Geometry: see drawing. Coordinates: mm, zero at the bounding-box minimum. A direction names the side the tool comes from. Give positions to 0.01 mm unless a question says otherwise; leave off trailing zeros. Loops run counter-clockwise (first coordinate to the right, second up) from the corner with the lowest first, then second, coordinate; pieces in that order, holes last. Notation, with made-up numbers: M 38,70.25 L 48,70.25 A5 cw 48,76.25 Z; hole C 11,36 d1. An arc over 180 degrees is marked long. Answer in a Markdown table with one row per item.
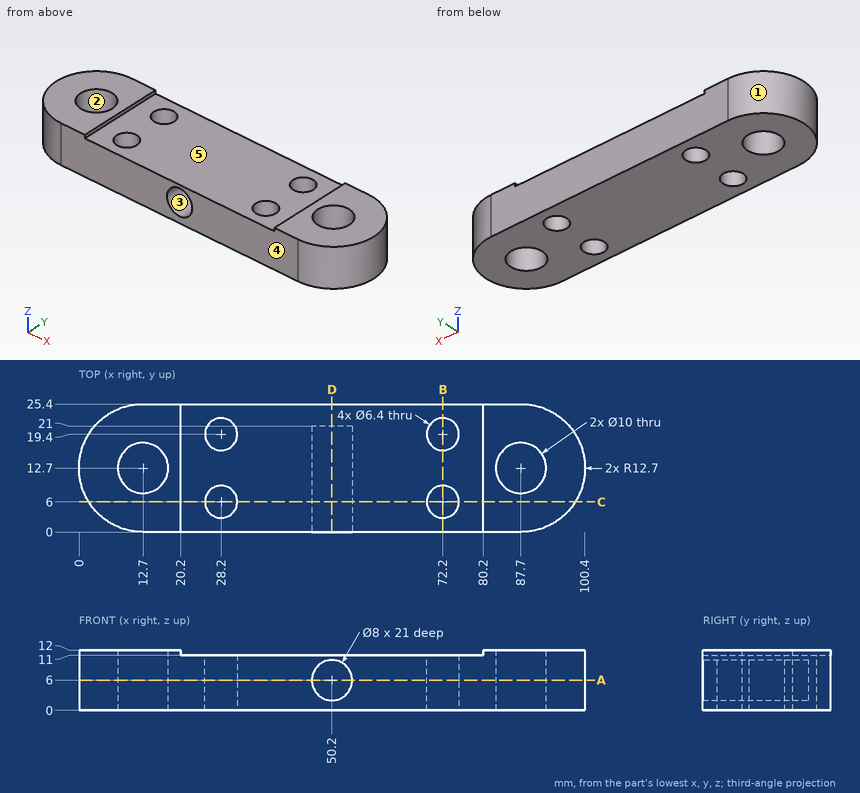
1) Section C-C, the plane y = 6. Return loops of the section in (x, z), then the cut area to 3 significant figures.
Reply:
| item | result |
|---|---|
| outline | M 1.91,0 L 25,0 L 25,11 L 20.2,11 L 20.2,12 L 1.91,12 Z; M 31.4,0 L 69,0 L 69,11 L 31.4,11 Z; M 75.4,0 L 98.49,0 L 98.49,12 L 80.2,12 L 80.2,11 L 75.4,11 Z; hole C 50.2,6 d8 |
| area | 908 mm² |
2) Section A-A, the plane z = 6. Return loops of the section in (x, y), then the cut area to 3 significant figures.
Reply:
| item | result |
|---|---|
| outline | M 12.7,0 L 46.2,0 L 46.2,21 L 54.2,21 L 54.2,0 L 87.7,0 A12.7 ccw 87.7,25.4 L 12.7,25.4 A12.7 ccw Z; hole C 12.7,12.7 d10; hole C 28.2,6 d6.4; hole C 28.2,19.4 d6.4; hole C 72.2,6 d6.4; hole C 72.2,19.4 d6.4; hole C 87.7,12.7 d10 |
| area | 1,960 mm² |
3) Section B-B, the plane x = 72.2. Return loops of the section in (y, z), then the cut area to 3 significant figures.
Reply:
| item | result |
|---|---|
| outline | M 0,0 L 2.8,0 L 2.8,11 L 0,11 Z; M 9.2,0 L 16.2,0 L 16.2,11 L 9.2,11 Z; M 22.6,0 L 25.4,0 L 25.4,11 L 22.6,11 Z |
| area | 139 mm² |
4) Set-up query: the marked faces 4 and 5. Return all of +Z, -Z, +X, -X, +Y, -Y with unobstructed straight access to the full face (end or side cutting, diameter ignored); none if empty.
Reply:
| item | result |
|---|---|
| face 4 | +Z, -Z, +X, -X, -Y |
| face 5 | +Z, +Y, -Y |
5) Pin query (flat end, axial travel): pin 1 Ø10 at (x, y) = (28.2, 19.4) entering from +Z; pin 2 Ø6.5 at (x, z) = (50.2, 6) entering from -Y; pin 3 Ø1.1 at (y, z) = (18.5, 11.5) entering from +X. Return the tip coordinate at first contact, or that it passes through.
Reply:
| item | result |
|---|---|
| pin 1 | stops at z = 11 |
| pin 2 | stops at y = 21 |
| pin 3 | stops at x = 99.26 |
6) Section D-D, the plane x = 50.2. Return loops of the section in (y, z).
Reply:
| item | result |
|---|---|
| outline | M 0,0 L 25.4,0 L 25.4,11 L 0,11 L 0,10 L 21,10 L 21,2 L 0,2 Z |
7) Material intervals for L1, parallel to Y at x = 28.2, z = 3; L2, parallel to X at y = 13.75, z = 7.75; L3, parallel to X at y = 15.5, z = 6, sorted ascending.
Reply:
| item | result |
|---|---|
| L1 | y = 0 to 2.8, 9.2 to 16.2, 22.6 to 25.4 |
| L2 | x = 0.04 to 7.81, 17.59 to 46.6, 53.8 to 82.81, 92.59 to 100.36 |
| L3 | x = 0.31 to 8.56, 16.84 to 46.2, 54.2 to 83.56, 91.84 to 100.09 |
8) Pull-direction query (Y, two-part tool) for the marked faces 1, 2 and 3; classes: released by +Y, released by -Y, zero draft, split by the parting line, or undercut.
Reply:
| item | result |
|---|---|
| face 1 | split by the parting line |
| face 2 | undercut |
| face 3 | zero draft |
